from build123d import *

# Parameters (mm, degrees)
PLATE_START                   = 28.55
PLATE_D_DEPTH                 = 6
BOX_START                     = -28.55
SKETCH2_W                     = 3.5
SKETCH2_H                     = 28
BOX_WALLS_DEPTH               = 57.3
WALL_START                    = -28.55
SKETCH3_W                     = 3.5
SKETCH3_H                     = 10
WALL_BOSSES_DEPTH             = 57.3
HORN_START                    = 28.35
HORN_POCKET_DEPTH             = 2.5
BOLT_START                    = 28.35
SKETCH5_R                     = 1.7
BOLT_HOLES_DEPTH              = 6.4
HUB_START                     = 32.05
SKETCH6_R                     = 3.2
HUB_COUNTERBORE_DEPTH         = 2.7
HEAD_MOUNT_START              = 31.55
SKETCH7_R                     = 3.2
HEAD_MOUNT_COUNTERBORES_DEPTH = 3.2
COVER_START                   = -28.75
SKETCH8_R                     = 1.7
COVER_BOLT_HOLES_DEPTH        = 10.2
COVER_START_2                 = -24.9
COVER_NUT_SLOTS_OUTLINE_R     = 1.7
COVER_NUT_SLOTS_DEPTH         = 2.7


with BuildPart() as part:
    # Sketch1 → Plate D (new body)
    with BuildSketch(Plane(origin=(0, 0, 0), x_dir=(0, 0, -1), z_dir=(1, 0, 0)).offset(PLATE_START)):
        with BuildLine():
            Line((-32, 227.975478406), (-32, 288.5))
            ThreePointArc((-32, 288.5), (-30.828427125, 291.328427125), (-28, 292.5))
            Line((-28, 292.5), (0, 292.5))
            ThreePointArc((0, 292.5), (2.828427125, 291.328427125), (4, 288.5))
            Line((4, 288.5), (4, 227.975478406))
            ThreePointArc((4, 227.975478406), (4.49156491, 225.597003504), (5.885714286, 223.608253536))
            ThreePointArc((5.885714286, 223.608253536), (-14, 173.5), (-33.885714286, 223.608253536))
            ThreePointArc((-33.885714286, 223.608253536), (-32.49156491, 225.597003504), (-32, 227.975478406))
        make_face()
    extrude(amount=PLATE_D_DEPTH)

    # Sketch2 → Box walls (add)
    with BuildSketch(Plane(origin=(0, 0, 0), x_dir=(0, 0, -1), z_dir=(1, 0, 0)).offset(BOX_START)):
        with Locations((2.25, 252.5)):
            Rectangle(SKETCH2_W, SKETCH2_H)
        with Locations((-30.25, 252.5)):
            Rectangle(SKETCH2_W, SKETCH2_H)
    extrude(amount=BOX_WALLS_DEPTH)

    # Sketch3 → Wall bosses (add)
    with BuildSketch(Plane(origin=(0, 0, 0), x_dir=(0, 0, -1), z_dir=(1, 0, 0)).offset(WALL_START)):
        with Locations((-1.25, 244.5)):
            Rectangle(SKETCH3_W, SKETCH3_H)
        with Locations((-26.75, 244.5)):
            Rectangle(SKETCH3_W, SKETCH3_H)
        with Locations((-1.25, 260.5)):
            Rectangle(SKETCH3_W, SKETCH3_H)
        with Locations((-26.75, 260.5)):
            Rectangle(SKETCH3_W, SKETCH3_H)
    extrude(amount=WALL_BOSSES_DEPTH)

    # Sketch4 → Horn pocket (cut)
    with BuildSketch(Plane(origin=(0, 0, 0), x_dir=(0, 0, -1), z_dir=(1, 0, 0)).offset(HORN_START)):
        with BuildLine():
            Line((-18.4, 179.4), (-18.4, 225.6))
            ThreePointArc((-18.4, 225.6), (-14, 230), (-9.6, 225.6))
            Line((-9.6, 225.6), (-9.6, 179.4))
            ThreePointArc((-9.6, 179.4), (-14, 175), (-18.4, 179.4))
        make_face()
    extrude(amount=HORN_POCKET_DEPTH, mode=Mode.SUBTRACT)

    # Sketch5 → Bolt holes (cut)
    with BuildSketch(Plane(origin=(0, 0, 0), x_dir=(0, 0, -1), z_dir=(1, 0, 0)).offset(BOLT_START)):
        with Locations(Location((-14, 202.5, 0), (0, 0, 180))):
            Circle(SKETCH5_R)
        with Locations((-7, 274.5)):
            Circle(SKETCH5_R)
        with Locations((-21, 274.5)):
            Circle(SKETCH5_R)
    extrude(amount=BOLT_HOLES_DEPTH, mode=Mode.SUBTRACT)

    # Sketch6 → Hub counterbore (cut)
    with BuildSketch(Plane(origin=(0, 0, 0), x_dir=(0, 0, -1), z_dir=(1, 0, 0)).offset(HUB_START)):
        with Locations((-14, 202.5)):
            Circle(SKETCH6_R)
    extrude(amount=HUB_COUNTERBORE_DEPTH, mode=Mode.SUBTRACT)

    # Sketch7 → Head-mount counterbores (cut)
    with BuildSketch(Plane(origin=(0, 0, 0), x_dir=(0, 0, -1), z_dir=(1, 0, 0)).offset(HEAD_MOUNT_START)):
        with Locations((-7, 274.5)):
            Circle(SKETCH7_R)
        with Locations((-21, 274.5)):
            Circle(SKETCH7_R)
    extrude(amount=HEAD_MOUNT_COUNTERBORES_DEPTH, mode=Mode.SUBTRACT)

    # Sketch8 → Cover bolt holes (cut)
    with BuildSketch(Plane(origin=(0, 0, 0), x_dir=(0, 0, -1), z_dir=(1, 0, 0)).offset(COVER_START)):
        with Locations(Location((0, 244.5, 0), (0, 0, 180))):
            Circle(SKETCH8_R)
        with Locations((-28, 244.5)):
            Circle(SKETCH8_R)
        with Locations(Location((0, 260.5, 0), (0, 0, 180))):
            Circle(SKETCH8_R)
        with Locations((-28, 260.5)):
            Circle(SKETCH8_R)
    extrude(amount=COVER_BOLT_HOLES_DEPTH, mode=Mode.SUBTRACT)

    # Cover nut slots: read off the stored shape, not the designer's step
    # Cover nut slots outline → Cover nut slots (cut)
    # profile 1 of 4: a face of its own
    with BuildSketch(Plane(origin=(0, 0, 0), x_dir=(0, 0, -1), z_dir=(1, 0, 0)).offset(COVER_START_2)):
        Polygon((-25, 247.45), (-29.703183294, 247.45), (-31.406366588, 244.5), (-29.703183294, 241.55), (-25, 241.55), align=None)
        with Locations((-28, 244.5)):
            Circle(COVER_NUT_SLOTS_OUTLINE_R, mode=Mode.SUBTRACT)
    # profile 2 of 4: a face of its own
    with BuildSketch(Plane(origin=(0, 0, 0), x_dir=(0, 0, -1), z_dir=(1, 0, 0)).offset(COVER_START_2)):
        Polygon((1.703183294, 247.45), (-3, 247.45), (-3, 241.55), (1.703183294, 241.55), (3.406366588, 244.5), align=None)
        with Locations((0, 244.5)):
            Circle(COVER_NUT_SLOTS_OUTLINE_R, mode=Mode.SUBTRACT)
    # profile 3 of 4: a face of its own
    with BuildSketch(Plane(origin=(0, 0, 0), x_dir=(0, 0, -1), z_dir=(1, 0, 0)).offset(COVER_START_2)):
        Polygon((-25, 263.45), (-29.703183294, 263.45), (-31.406366588, 260.5), (-29.703183294, 257.55), (-25, 257.55), align=None)
        with Locations((-28, 260.5)):
            Circle(COVER_NUT_SLOTS_OUTLINE_R, mode=Mode.SUBTRACT)
    # profile 4 of 4: a face of its own
    with BuildSketch(Plane(origin=(0, 0, 0), x_dir=(0, 0, -1), z_dir=(1, 0, 0)).offset(COVER_START_2)):
        Polygon((1.703183294, 263.45), (-3, 263.45), (-3, 257.55), (1.703183294, 257.55), (3.406366588, 260.5), align=None)
        with Locations((0, 260.5)):
            Circle(COVER_NUT_SLOTS_OUTLINE_R, mode=Mode.SUBTRACT)
    extrude(amount=COVER_NUT_SLOTS_DEPTH, mode=Mode.SUBTRACT)


solid = part.part
Here's how the part is built. I have some questions about the finished solid (model axes, mm). A direction names the side the tool comes from. Round coordinates to 2 decimals unless told otherwise and drop trailing zeros. Loops run counter-clockwise (first coordinate to the right, second up) from the corner with the lowest first, then second, coordinate; pieces in that order, holes last. Notation, with made-up numbers: (18, 26.5) - (35, 26.5) arc R5 ccw to (35, 35.5) - close; hole circle Ø5 at (-35, 52.5). An arc over 180 degrees is marked (long way). One line per question, with ' | ' between items. Start each with the question number.
Q1. I want a section at D-D (y = 274.5). Write out the boundary of the cut face in (x, z), then the cut area to 3 significant figures.
Q2. I want a section at C-C (y = 202.5). Write out the boundary of the cut face in (x, z), then the cut area to 3 significant figures.
Q3. Please list where these lines run through material, in increasing order: line 1 (Y direction, x = -20, z = 0); line 2 (Z direction, x = -27.5, y = 244.5); line 3 (Z direction, x = -12.5, y = 247). Write a range as [from, to].
Q4. For faces 4 (the cylindrical face through (30, 230, 14)), 5 (the flat face through (0, 239.5, 27)), 6 (the flat face through (0, 244, 3)), which set-ups out of +Z, -Z, +X, -X, +Y, -Y let a thin tool reach every point of the face, with its end or its side?
Q5. We'd pull the mould along Y, two halves only. Please class faces 1 (the flat face through (0, 239.5, 1)), 2 (the cylindrical face through (-20.401, 262.186, 28.221)), 3 (the cylindrical face through (31.508, 225.628, -4.478)): +Y half, -Y half, draft (parallel to the pull), parting line (faces both ways), or undercut.
Q6. Will these pins go through, and if not, where does the flat tip stop? pin 1 (2.5 mm diameter, centred on y = 260.5, z = 0, fed in from -X); pin 2 (5.5 mm diameter, centred on y = 274.5, z = 7, fed in from -X); pin 3 (1.5 mm diameter, centred on x = 6, z = -1.5, fed in from -Y); pin 4 (1.9 mm diameter, centred on y = 202, z = 13.5, fed in from +X).
Q7. I want a section at B-B (x = 6). Write out the boundary of the cut face in (y, z).
Q8. I want a section at A-A (z = 14). Write out the boundary of the cut face in (x, y).
Response values:
1) outline: (28.55, -4) - (34.55, -4) - (34.55, 3.8) - (31.55, 3.8) - (31.55, 5.3) - (28.55, 5.3) - close; (28.55, 8.7) - (31.55, 8.7) - (31.55, 10.2) - (34.55, 10.2) - (34.55, 17.8) - (31.55, 17.8) - (31.55, 19.3) - (28.55, 19.3) - close; (28.55, 22.7) - (31.55, 22.7) - (31.55, 24.2) - (34.55, 24.2) - (34.55, 32) - (28.55, 32) - close | area: 157 mm²
2) outline: (28.55, -15) - (34.55, -15) - (34.55, 10.8) - (32.05, 10.8) - (32.05, 12.3) - (30.85, 12.3) - (30.85, 9.6) - (28.55, 9.6) - close; (28.55, 18.4) - (30.85, 18.4) - (30.85, 15.7) - (32.05, 15.7) - (32.05, 17.2) - (34.55, 17.2) - (34.55, 43) - (28.55, 43) - close | area: 308 mm²
3) line 1: y = [239.5, 242.8], [246.2, 249.5], [255.5, 258.8], [262.2, 265.5] | line 2: z = [-4, -1.7], [1.7, 3], [25, 26.3], [29.7, 32] | line 3: z = [-4, 3], [25, 32]
4) face 4: -X | face 5: -X, -Y | face 6: -X, +Y, -Y
5) face 1: -Y half | face 2: undercut | face 3: +Y half
6) pin 1: stops at x = -18.55 | pin 2: stops at x = 28.55 | pin 3: stops at y = 238.5 | pin 4: passes through
7) outline: (238.5, -4) - (266.5, -4) - (266.5, -0.5) - (265.5, -0.5) - (265.5, 3) - (255.5, 3) - (255.5, -0.5) - (249.5, -0.5) - (249.5, 3) - (239.5, 3) - (239.5, -0.5) - (238.5, -0.5) - close; (238.5, 28.5) - (239.5, 28.5) - (239.5, 25) - (249.5, 25) - (249.5, 28.5) - (255.5, 28.5) - (255.5, 25) - (265.5, 25) - (265.5, 28.5) - (266.5, 28.5) - (266.5, 32) - (238.5, 32) - close
8) outline: (28.55, 173.5) - (34.55, 173.5) - (34.55, 199.3) - (32.05, 199.3) - (32.05, 200.8) - (30.85, 200.8) - (30.85, 175) - (28.55, 175) - close; (28.55, 230) - (30.85, 230) - (30.85, 204.2) - (32.05, 204.2) - (32.05, 205.7) - (34.55, 205.7) - (34.55, 292.5) - (28.55, 292.5) - close
